Geometry check sheet. Reference: the model listing, model coordinates, mm. Face numbers are marked on the shaded views. A direction names the side the tool comes from. Round coordinates to 2 decimals unless told otherwise and drop trailing zeros. Write each loop counter-clockwise with the first axis right and the second up, starting at its lowest first coordinate (ties: lowest second). Pieces come first, ordered by that corner, then holes.
Item 1: Scan lines: probe 1 along X at (y, z) = (8.5, -5.5); probe 2 along Y at (x, z) = (0.25, 0); probe 3 along Z at (x, y) = (-3.75, 2). Record each from-to range of solid material in increasing order.
Item 2: Access from +Z, -Z, +X, -X, +Y, -Y to the whole of each face (thin tool, end or side, straight path). Record for the marked faces 5, 6 and 7.
Item 3: Cross-section at A-A (y = 5). Enter the section's corners in (x, z), then the cut area to 3 significant figures.
Item 4: Draft check along Z on the marked faces 1, 2, 3 and 4. Enter one of: pulls with the +Z half, pulls with the -Z half, needs draft (parallel to the pull), parting line crosses it, or undercut.
Item 5: Cross-section at C-C (z = 0). Enter the section's corners in (x, y).
Item 6: Cross-section at B-B (x = -1.75). Enter the section's corners in (y, z), then the cut area to 3 significant figures.
Item 7: Cross-section at D-D (z = 3.75). Enter the section's corners in (x, y), then the cut area to 3 significant figures.
Item 8: Depth check by flat-ended pin: P1, Ø1.5, axis at y = 6.5, z = 3, coming from the -X side; P2, Ø6, axis at x = 0, y = -2.5, coming from the -Z side; P3, Ø4, axis at y = 5, z = 0, coming from the +X side; P4, Ø1.5, axis at y = -15, z = 1, coming from the -X side. Enter the tip coordinate at first touch or a pass-through.
from build123d import *

# Parameters (mm, degrees)
SKETCH_1_W          = 7.56
SKETCH_1_H          = 12.56
EXTRUDE_1_DEPTH     = 10
CHAMFER_1_SIZE      = 1
EXTRUDE_2_DEPTH     = 5
SKETCH_4_R          = 1.45
CUT_EXTRUDE_1_DEPTH = 10
FILLET_1_R          = 1


with BuildPart() as part:
    # ｽｹｯﾁ1 → ﾎﾞｽ - 押し出し1 (new body)
    with BuildSketch(Plane(origin=(0, 0, 0), x_dir=(1, 0, 0), z_dir=(0, 1, 0))):
        Rectangle(SKETCH_1_W, SKETCH_1_H)
    extrude(amount=EXTRUDE_1_DEPTH)

    # 面取り1
    chamfer_1_edges = [part.edges().sort_by_distance(p)[0] for p in [
        (3.78, 10, 0),
        (0, 10, -6.28),
        (-3.78, 10, 0),
        (0, 10, 6.28),
    ]]
    chamfer(chamfer_1_edges, length=CHAMFER_1_SIZE)

    # ｽｹｯﾁ3 → ﾎﾞｽ - 押し出し2 (add, symmetric)
    with BuildSketch(Plane(origin=(0, 0, 0), x_dir=(0, 0, -1), z_dir=(1, 0, 0))):
        Polygon((0, 0), (-6.28, 0), (-7.5, 0), (-7.5, -25.980762114), (7.5, 0), (6.28, 0), align=None)
    extrude(amount=EXTRUDE_2_DEPTH, both=True)

    # ｽｹｯﾁ4 → ｶｯﾄ - 押し出し1 (cut)
    with BuildSketch(Plane(origin=(3.78, 0, 0), x_dir=(0, 0, -1), z_dir=(1, 0, 0))):
        with Locations((0, 5)):
            Circle(SKETCH_4_R)
    extrude(amount=-CUT_EXTRUDE_1_DEPTH, mode=Mode.SUBTRACT)

    # ﾌｨﾚｯﾄ1
    fillet_1_edges = [part.edges().sort_by_distance(p)[0] for p in [
        (0, -25.980762114, 7.5),
    ]]
    fillet(fillet_1_edges, radius=FILLET_1_R)


solid = part.part
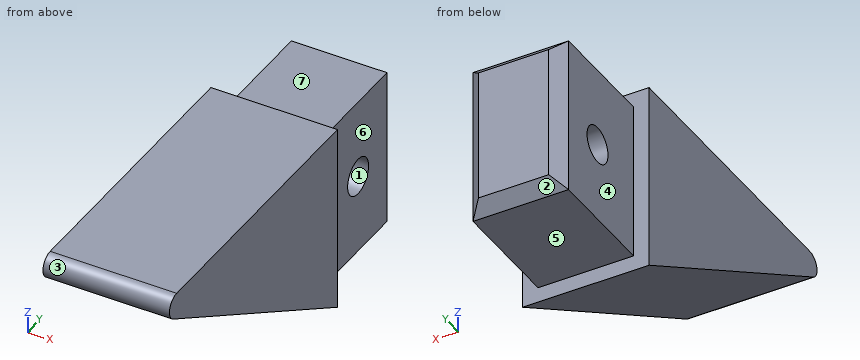
Resolved:
1. probe 1: x = -3.78 to 3.78
1. probe 2: y = -12.99 to 3.55, 6.45 to 10
1. probe 3: z = -6.28 to 6.28
2. face 5: -Z, +X, -X, +Y
2. face 6: +Z, -Z, +X, +Y
2. face 7: +Z, +X, -X, +Y
3. outline: (-3.78, -6.28) - (3.78, -6.28) - (3.78, -1.45) - (-3.78, -1.45) - close; (-3.78, 1.45) - (3.78, 1.45) - (3.78, 6.28) - (-3.78, 6.28) - close
3. area: 73.0 mm2
4. face 1: undercut
4. face 2: pulls with the -Z half
4. face 3: parting line crosses it
4. face 4: needs draft
5. outline: (-5, -12.99) - (5, -12.99) - (5, 0) - (3.78, 0) - (3.78, 3.55) - (-3.78, 3.55) - (-3.78, 0) - (-5, 0) - close; (-3.78, 6.45) - (3.78, 6.45) - (3.78, 9) - (2.78, 10) - (-2.78, 10) - (-3.78, 9) - close
6. outline: (-22.75, 5.63) - (0, -7.5) - (0, -6.28) - (9, -6.28) - (10, -5.28) - (10, 5.28) - (9, 6.28) - (0, 6.28) - (0, 7.5) - (-22.25, 7.5) arc R1 ccw to start; hole circle Ø2.9 at (5, 0)
6. area: 310 mm2
7. outline: (-5, -19.49) - (5, -19.49) - (5, 0) - (3.78, 0) - (3.78, 9) - (2.78, 10) - (-2.78, 10) - (-3.78, 9) - (-3.78, 0) - (-5, 0) - close
7. area: 269 mm2
8. P1: stops at x = -3.78
8. P2: stops at z = -7.5
8. P3: stops at x = 3.78
8. P4: stops at x = -5
